The model under review builds one solid part; all positions refer to its coordinate system, in mm. Face numbers are marked on the shaded views. A direction names the side the tool comes from. Round coordinates to 2 decimals unless told otherwise and drop trailing zeros. Loops run counter-clockwise (first coordinate to the right, second up) from the corner with the lowest first, then second, coordinate; pieces in that order, holes last. Notation, with made-up numbers: M 70,-29.75 L 117,-29.75 A22 ccw 117,-20.75 Z; hole C -9.5,-9 d9. An arc over 180 degrees is marked long. Return JSON: item names as keys, results as strings. Group by question number.
Q1. Draft analysis for pull direction Z (two halves, no side actions). For the marked faces 1, 2 and 3, state which applies: pulls with the +Z half, pulls with the -Z half, needs draft (parallel to the pull), parting line crosses it, or undercut.
Q2. Consider section B-B (z = 0). State the section outline as (x, y) points.
Q3. Consider section C-C (y = -15). State the section outline as (x, z) points, and give its area (4 significant figures).
Q4. To check wall thickness, follow line 1 along Y through (x, z) = (-2, 0.25); line 2 along Y through (x, z) = (1, 11.75); line 3 along X through (y, z) = (12, -10.75). State the ranges of each line that lie inside material, in increasing order.
Q5. Consider section A-A (x = 1.75). State the section outline as (y, z) points.
Q6. Consider section D-D (z = -7.75). State the section outline as (x, y) points.
Q7. For the marked faces 4 and 5, list the 3-axis set-ups (+Z, -Z, +X, -X, +Y, -Y) from which the entire face can be reached by the end or side of a thin tool; tool diameter is ignored.
Q8. Clearance check with a flat-ended pin moving along its axis: pin 1 Ø9 at (y, z) = (15, 0) entering from +X. State where the tip first meets the part, or that it passes through.
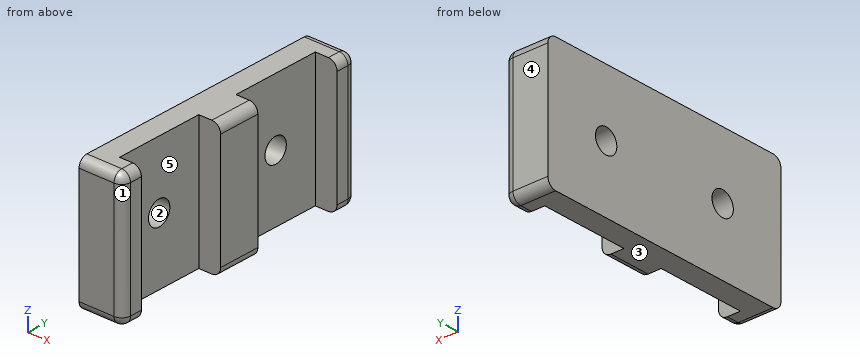
from build123d import *

# Parameters (mm, degrees)
SKETCH_2_R      = 2.75
EXTRUDE_1_DEPTH = 5
EXTRUDE_START   = 5
SKETCH_4_W      = 30
SKETCH_4_H      = 9.6
EXTRUDE_2_DEPTH = 5
FILLET_1_R      = 2


with BuildPart() as part:
    # ｽｹｯﾁ2 → ﾎﾞｽ - 押し出し1 (new body)
    with BuildSketch(Plane(origin=(0, 0, 0), x_dir=(0, 0, -1), z_dir=(1, 0, 0))):
        with BuildLine():
            Line((-15, 28), (-15, -28))
            ThreePointArc((-15, -28), (-14.414213562, -29.414213562), (-13, -30))
            Line((-13, -30), (13, -30))
            ThreePointArc((13, -30), (14.414213562, -29.414213562), (15, -28))
            Line((15, -28), (15, 28))
            ThreePointArc((15, 28), (14.414213562, 29.414213562), (13, 30))
            Line((13, 30), (-13, 30))
            ThreePointArc((-13, 30), (-14.414213562, 29.414213562), (-15, 28))
        make_face()
        with Locations((0, 15)):
            Circle(SKETCH_2_R, mode=Mode.SUBTRACT)
        with Locations((0, -15)):
            Circle(SKETCH_2_R, mode=Mode.SUBTRACT)
    extrude(amount=-EXTRUDE_1_DEPTH)

    # ｽｹｯﾁ4 → ﾎﾞｽ - 押し出し2 (add)
    with BuildSketch(Plane(origin=(0, 0, 0), x_dir=(0, 0, -1), z_dir=(1, 0, 0)).offset(EXTRUDE_START)):
        with BuildLine():
            Line((-15, 28), (-15, 25.2))
            Line((-15, 25.2), (15, 25.2))
            Line((15, 25.2), (15, 28))
            ThreePointArc((15, 28), (14.414213562, 29.414213562), (13, 30))
            Line((13, 30), (-13, 30))
            ThreePointArc((-13, 30), (-14.414213562, 29.414213562), (-15, 28))
        make_face()
        Rectangle(SKETCH_4_W, SKETCH_4_H)
        with BuildLine():
            Line((15, -25.2), (-15, -25.2))
            Line((-15, -25.2), (-15, -28))
            ThreePointArc((-15, -28), (-14.414213562, -29.414213562), (-13, -30))
            Line((-13, -30), (13, -30))
            ThreePointArc((13, -30), (14.414213562, -29.414213562), (15, -28))
            Line((15, -28), (15, -25.2))
        make_face()
    extrude(amount=-EXTRUDE_2_DEPTH)

    # ﾌｨﾚｯﾄ1
    fillet_1_edges = [part.edges().sort_by_distance(p)[0] for p in [
        (5, 26.6, 15),
        (5, 26.6, -15),
        (5, 29.414213562, -14.414213562),
        (5, 30, 0),
        (5, 29.414213562, 14.414213562),
        (5, 0, -15),
        (5, 0, 15),
        (5, -26.6, -15),
        (5, -26.6, 15),
        (5, -29.414213562, 14.414213562),
        (5, -30, 0),
        (5, -29.414213562, -14.414213562),
    ]]
    fillet(fillet_1_edges, radius=FILLET_1_R)


solid = part.part
Values:
{
 "1": {"face 1": "needs draft", "face 2": "undercut", "face 3": "pulls with the -Z half"},
 "2": {"outline": "M -5,-30 L 3,-30 A2 ccw 5,-28 L 5,-25.2 L 0,-25.2 L 0,-17.75 L -5,-17.75 Z; M -5,-12.25 L 0,-12.25 L 0,-4.8 L 5,-4.8 L 5,4.8 L 0,4.8 L 0,12.25 L -5,12.25 Z; M -5,17.75 L 0,17.75 L 0,25.2 L 5,25.2 L 5,28 A2 ccw 3,30 L -5,30 Z"},
 "3": {"outline": "M -5,-15 L 0,-15 L 0,-2.75 L -5,-2.75 Z; M -5,2.75 L 0,2.75 L 0,15 L -5,15 Z", "area": "122.5 mm2"},
 "4": {"line 1": "y = -30 to -17.74, -12.26 to 12.26, 17.74 to 30", "line 2": "y = -30 to -25.2, -4.8 to 4.8, 25.2 to 30", "line 3": "x = -5 to 0"},
 "5": {"outline": "M -30,-13 A2 ccw -28,-15 L -25.2,-15 L -25.2,15 L -28,15 A2 ccw -30,13 Z; M -4.8,-15 L 4.8,-15 L 4.8,15 L -4.8,15 Z; M 25.2,-15 L 28,-15 A2 ccw 30,-13 L 30,13 A2 ccw 28,15 L 25.2,15 Z"},
 "6": {"outline": "M -5,-30 L 3,-30 A2 ccw 5,-28 L 5,-25.2 L 0,-25.2 L 0,-4.8 L 5,-4.8 L 5,4.8 L 0,4.8 L 0,25.2 L 5,25.2 L 5,28 A2 ccw 3,30 L -5,30 Z"},
 "7": {"face 4": "+Z, -Z, +X, -X, +Y", "face 5": "+Z, -Z, +X"},
 "8": {"pin 1": "stops at x = 0"}
}
